from build123d import *

# Parameters (mm, degrees)
SKETCH1_W                                           = 100
SKETCH1_H                                           = 100
BOSS_EXTRUDE1_DEPTH                                 = 12.7
M5_CLEARANCE_HOLE1_D                                = 6.06
CSK_FOR_3_8_FLAT_HEAD_SOCKET_CAP_SCREW1_D           = 10.0838
CSK_FOR_3_8_FLAT_HEAD_SOCKET_CAP_SCREW1_CSINK_D     = 19.8374
CSK_FOR_3_8_FLAT_HEAD_SOCKET_CAP_SCREW1_CSINK_ANGLE = 82


with BuildPart() as part:
    # Sketch1 → Boss-Extrude1 (new body)
    with BuildSketch(Plane(origin=(0, 0, 0), x_dir=(1, 0, 0), z_dir=(0, 1, 0))):
        with Locations((0, 10)):
            Rectangle(SKETCH1_W, SKETCH1_H)
    extrude(amount=BOSS_EXTRUDE1_DEPTH)

    # M5 Clearance Hole1 (through all)
    with Locations(Plane(origin=(0, 12.7, 0), x_dir=(1, 0, 0), z_dir=(0, 1, 0))):
        with Locations((-40, 50), (40, 50), (40, -30), (-40, -30)):
            Hole(M5_CLEARANCE_HOLE1_D / 2)

    # CSK for 3/8 Flat Head Socket Cap Screw1 (through all)
    with Locations(Plane(origin=(0, 0, 0), x_dir=(-1, 0, 0), z_dir=(0, -1, 0))):
        with Locations((0, 0)):
            CounterSinkHole(CSK_FOR_3_8_FLAT_HEAD_SOCKET_CAP_SCREW1_D / 2, CSK_FOR_3_8_FLAT_HEAD_SOCKET_CAP_SCREW1_CSINK_D / 2, counter_sink_angle=CSK_FOR_3_8_FLAT_HEAD_SOCKET_CAP_SCREW1_CSINK_ANGLE)


solid = part.part
The model under review builds one solid part; all positions refer to its coordinate system, in mm. Round coordinates to 2 decimals unless told otherwise and drop trailing zeros. Loops run counter-clockwise (first coordinate to the right, second up) from the corner with the lowest first, then second, coordinate; pieces in that order, holes last. Notation, with made-up numbers: (-13.5, -21.75) -> (11.5, -21.75) arc R18 ccw to (11.5, -14.75) -> close; hole circle Ø7 at (4, 87.5). An arc over 180 degrees is marked (long way). Answer as CSV lines item,"result".
1) To check wall thickness, follow line 1 along Z through (x, y) = (40, 9.5); line 2 along X through (y, z) = (4.75, -50); line 3 along Z through (x, y) = (0, 10). State the ranges of each line that lie inside material, in increasing order. Write a range as from..to.
Geometry results:
line 1,"z = -60..-53.03, -46.97..26.97, 33.03..40"
line 2,"x = -50..-43.03, -36.97..36.97, 43.03..50"
line 3,"z = -60..-5.04, 5.04..40"
2) Add section C-C on x = 0. Write out the cut boundary in (y, z).
Geometry results:
outline,"(0, -60) -> (12.7, -60) -> (12.7, -5.04) -> (5.61, -5.04) -> (0, -9.92) -> close; (0, 9.92) -> (5.61, 5.04) -> (12.7, 5.04) -> (12.7, 40) -> (0, 40) -> close"
3) Draft analysis for pull direction Z (two halves, no side actions). For faces 1 (the face through (-0.66, 9.2, -5)), 2 (the face through (-1, 6, 40)), 3 (the face through (-50, 6, -9)), state which applies: pulls with the +Z half, pulls with the -Z half, needs draft (parallel to the pull), parting line crosses it, or undercut.
Geometry results:
face 1,"undercut"
face 2,"pulls with the +Z half"
face 3,"needs draft"
4) For P1, Ø3.5, axis at x = 40, z = 30, coming from the +Y side; P2, Ø10, axis at x = -33, z = 14, coming from the -Y side, all flat-tipped, find the tip position at first contact; note any pin that passes through.
Geometry results:
P1,"passes through"
P2,"stops at y = 0"
5) Add section D-D on x = 40. Write out the cut boundary in (y, z), plus the area to 3 significant figures.
Geometry results:
outline,"(0, -60) -> (12.7, -60) -> (12.7, -53.03) -> (0, -53.03) -> close; (0, -46.97) -> (12.7, -46.97) -> (12.7, 26.97) -> (0, 26.97) -> close; (0, 33.03) -> (12.7, 33.03) -> (12.7, 40) -> (0, 40) -> close"
area,"1,120 mm²"
6) Add section A-A on z = -50. Write out the cut boundary in (x, y), plus the area to 3 significant figures.
Geometry results:
outline,"(-50, 0) -> (-43.03, 0) -> (-43.03, 12.7) -> (-50, 12.7) -> close; (-36.97, 0) -> (36.97, 0) -> (36.97, 12.7) -> (-36.97, 12.7) -> close; (43.03, 0) -> (50, 0) -> (50, 12.7) -> (43.03, 12.7) -> close"
area,"1,120 mm²"
7) Add section B-B on y = 11.5. Write out the cut boundary in (x, z).
Geometry results:
outline,"(-50, -60) -> (50, -60) -> (50, 40) -> (-50, 40) -> close; hole circle Ø6.06 at (-40, -50); hole circle Ø6.06 at (-40, 30); hole circle Ø10.08 at (0, 0); hole circle Ø6.06 at (40, -50); hole circle Ø6.06 at (40, 30)"
